Read the model definition and answer for the solid it produces. Units are mm, in the model's axes. Round coordinates to 2 decimals unless told otherwise and drop trailing zeros. Write each loop counter-clockwise with the first axis right and the second up, starting at its lowest first coordinate (ties: lowest second). Pieces come first, ordered by that corner, then holes. Notation, with made-up numbers: (48.25, 71.25) - (92.25, 71.25) arc R26 cw to (92.25, 87.25) - close; hole circle Ø1 at (18, -38.5). An arc over 180 degrees is marked (long way). Use one line per item in the form item = value. Start each with the question number.
1) For a pull along X with two mould halves and no side action, classify faces 1 (the face through (60.92, 25.39, 35.6)), 2 (the face through (38.79, 25.76, 15.95)), 3 (the face through (0, 28, 19)) as released by +X, released by -X, zero draft, split by the parting line, or undercut.
2) The part is cut by section C-C, the plane x = 25.4. Give the vertices of the cut face in (y, z) (3 decimals), plus the area to 3 significant figures.
3) The part is cut by section A-A, the plane z = 25.4. Give the vertices of the cut face in (x, y) (3 decimals).
4) The part is cut by section B-B, the plane y = 30. Give the vertices of the cut face in (x, z) (3 decimals).
5) Consider line 1 along X through (y, z) = (31, 25); line 2 along X through (y, z) = (14, 23.5); line 3 along Z through (x, y) = (44, 36). Determine where each line is inside the solid, lowest interval first. Write a range as from..to.
from build123d import *

# Parameters (mm, degrees)
F0_W     = 63.5
F0_H     = 38.1
F1_DEPTH = 50.8
F2_SIZE  = 5.08
F3_R     = 5.08
F3_R_2   = 5.07999
F5_D     = 6.35


# Not quite as in the source:
# - a fillet or chamfer is up to 0.001 mm smaller than in the source, because OpenCascade refuses the exact size


with BuildPart() as f1:
    # F0 (on Front) → F1 (new body)
    with BuildSketch(Plane.XZ):
        with Locations((31.75, 19.05)):
            Rectangle(F0_W, F0_H)
    extrude(amount=-F1_DEPTH)

    # F2
    f2_edges = [f1.edges().sort_by_distance(p)[0] for p in [
        (63.5, 25.4, 38.1),
        (0, 25.4, 38.1),
        (63.5, 25.4, 0),
        (0, 25.4, 0),
    ]]
    chamfer(f2_edges, length=F2_SIZE)

    # F3 (call 1 of 4: OpenCascade refuses the feature's edges together)
    f3_edges = [f1.edges().sort_by_distance(p)[0] for p in [
        (63.5, 0, 19.05),
    ]]
    fillet(f3_edges, radius=F3_R)

    # F3#2 (call 2 of 4)
    f3_2_edges = [f1.edges().sort_by_distance(p)[0] for p in [
        (0, 0, 19.05),
    ]]
    fillet(f3_2_edges, radius=F3_R)

    # F3#3 (call 3 of 4) (radius 5.08 in the source; OpenCascade refuses exactly that, so slightly less here)
    f3_3_edges = [f1.edges().sort_by_distance(p)[0] for p in [
        (31.75, 0, 0),
    ]]
    fillet(f3_3_edges, radius=F3_R_2)

    # F3#4 (call 4 of 4) (radius 5.08 in the source; OpenCascade refuses exactly that, so slightly less here)
    f3_4_edges = [f1.edges().sort_by_distance(p)[0] for p in [
        (31.75, 0, 38.1),
    ]]
    fillet(f3_4_edges, radius=F3_R_2)

    # F5 (through all)
    with Locations(Plane.XZ):
        with Locations((25.4, 12.7), (44.45, 25.4), (38.1, 19.05)):
            Hole(F5_D / 2)


with BuildPart() as f6_1:
    # F6: copy of F1
    add(f1.part.moved(Location((50.8, 50.8, 50.8))))


solid = f1.part
Geometry results:
q1.face_1 = released by +X
q1.face_2 = undercut
q1.face_3 = released by -X
q2.outline = (0, 5.08) arc R5.08 ccw to (5.08, 0) - (50.8, 0) - (50.8, 9.525) - (0, 9.525) - close; (0, 15.875) - (50.8, 15.875) - (50.8, 38.1) - (5.08, 38.1) arc R5.08 ccw to (0, 33.02) - close
q2.area = 1,600 mm2
q3.outline = (0, 5.08) arc R5.08 ccw to (5.08, 0) - (41.275, 0) - (41.275, 50.8) - (0, 50.8) - close; (47.625, 0) - (58.42, 0) arc R5.08 ccw to (63.5, 5.08) - (63.5, 50.8) - (47.625, 50.8) - close
q4.outline = (0, 5.08) - (5.08, 0) - (58.42, 0) - (63.5, 5.08) - (63.5, 33.02) - (58.42, 38.1) - (5.08, 38.1) - (0, 33.02) - close; hole circle Ø6.35 at (25.4, 12.7); hole circle Ø6.35 at (38.1, 19.05); hole circle Ø6.35 at (44.45, 25.4)
q5.line_1 = 0..41.3, 47.6..63.5
q5.line_2 = 0..41.91, 46.99..63.5
q5.line_3 = 0..22.26, 28.54..38.1
